Autodesk Inventor part; units mm, degrees
ref_plane "YZ Plane" through (0, 0, 0) normal (1, 0, 0) x (0, 1, 0)
ref_plane "XZ Plane" through (0, 0, 0) normal (0, 1, 0) x (-1, 0, 0)
ref_plane "XY Plane" through (0, 0, 0) normal (0, 0, 1) x (1, 0, 0)
sketch "Sketch1" plane through (0, 0, 0) normal (0, 0, 1) x (1, 0, 0)
  line L0 (1.5, 0) -> (1.5, 9)
  line L1 (1.5, 9) -> (6.5, 9)
  line L2 (6.5, 9) -> (6.5, 7.5)
  line L3 (6.5, 7.5) -> (4.5, 7.5)
  line L4 (4.5, 7.5) -> (4.5, 1.5)
  line L5 (4.5, 1.5) -> (6.5, 1.5)
  line L6 (6.5, 1.5) -> (6.5, 0)
  line L7 (6.5, 0) -> (1.5, 0)
  line L8 (0, -1.8) -> (0, 10.8)
  point P0 (0, 0)
  dimension "d0" = 9
  dimension "d1" = 5
  dimension "d2" = 1.5
  dimension "d3" = 2
  dimension "d4" = 1.5
revolve "Revolution1" add sketch "Sketch1" angle 360 about axis through (0, -10, 0) along (0, 1, 0)
properties part number "IdlePulley"
Read the model definition and answer for the solid it produces. Units are mm, in the model's axes. A direction names the side the tool comes from. Coordinates: 2 decimals unless noted, no trailing zeros. Write each loop counter-clockwise with the first axis right and the second up, starting at its lowest first coordinate (ties: lowest second). Pieces come first, ordered by that corner, then holes. Notation, with made-up numbers: M 81.25,-5.5 L 97.25,-5.5 A33 ccw 97.25,31.5 Z; hole C -13.75,-25 d7. An arc over 180 degrees is marked long. Use a Markdown table: item, result.
Q1. Straight lines are drawn through the part: L1, parallel to Y at x = 4, z = -3.25; L2, parallel to X at y = 2, z = 0. For each, find the intervals that lie inside material, in ascending order. Write a range as [from, to].
Answer block:
| item | result |
|---|---|
| L1 | y = [0, 1.5], [7.5, 9] |
| L2 | x = [-4.5, -1.5], [1.5, 4.5] |
Q2. Which of the six approach directions +Z, -Z, +X, -X, +Y, -Y give full straight-line access (tool end or side, diameter ignored) to faces 1 (the face through (-5.158, 0.74, -3.955)), 2 (the face through (-1.54, 1.5, -4.42))?
Answer block:
| item | result |
|---|---|
| face 1 | +Y, -Y |
| face 2 | none |
Q3. The part is cut by section C-C, the plane y = 6.75. Write down the section's boundary in (x, z), then the cut area to 3 significant figures.
Answer block:
| item | result |
|---|---|
| outline | C 0,0 d9; hole C 0,0 d3 |
| area | 56.5 mm2 |
Q4. Each of these flat-tipped pins is pushed along its axis until it touches: pin 1 Ø3 at (y, z) = (2, 5) entering from +X; pin 2 Ø5 at (x, y) = (-3.5, 1.5) entering from +Z. Where does it stop, or does it pass through?
Answer block:
| item | result |
|---|---|
| pin 1 | stops at x = 5.42 |
| pin 2 | stops at z = 6.42 |
Q5. Determine the mould class of faces 3 (the face through (-0.59, 4.46, 4.46)), 4 (the face through (-1.5, 4.56, -0.07)), 5 (the face through (-1.54, 7.5, -4.42)) for opening direction Z: released by +Z, released by -Z, zero draft, split by the parting line, or undercut.
Answer block:
| item | result |
|---|---|
| face 3 | split by the parting line |
| face 4 | undercut |
| face 5 | zero draft |
Q6. The part is cut by section D-D, the plane x = -3. Write down the section's boundary in (y, z).
Answer block:
| item | result |
|---|---|
| outline | M 0,-5.77 L 1.5,-5.77 L 1.5,-3.35 L 7.5,-3.35 L 7.5,-5.77 L 9,-5.77 L 9,5.77 L 7.5,5.77 L 7.5,3.35 L 1.5,3.35 L 1.5,5.77 L 0,5.77 Z |
Q7. The part is cut by section A-A, the plane x = 0. Write down the section's boundary in (y, z), then the cut area to 3 significant figures.
Answer block:
| item | result |
|---|---|
| outline | M 0,-6.5 L 1.5,-6.5 L 1.5,-4.5 L 7.5,-4.5 L 7.5,-6.5 L 9,-6.5 L 9,-1.5 L 0,-1.5 Z; M 0,1.5 L 9,1.5 L 9,6.5 L 7.5,6.5 L 7.5,4.5 L 1.5,4.5 L 1.5,6.5 L 0,6.5 Z |
| area | 66.0 mm2 |
Q8. The part is cut by section B-B, the plane z = 0. Write down the section's boundary in (x, y), then the cut area to 3 significant figures.
Answer block:
| item | result |
|---|---|
| outline | M -6.5,0 L -1.5,0 L -1.5,9 L -6.5,9 L -6.5,7.5 L -4.5,7.5 L -4.5,1.5 L -6.5,1.5 Z; M 1.5,0 L 6.5,0 L 6.5,1.5 L 4.5,1.5 L 4.5,7.5 L 6.5,7.5 L 6.5,9 L 1.5,9 Z |
| area | 66.0 mm2 |
